from build123d import *

# Parameters (mm, degrees)
F0_R     = 10.428739
F1_DEPTH = 30


with BuildPart() as f1:
    # F0 (on Front) → F1 (new body)
    with BuildSketch(Plane.XZ):
        Polygon((-53.313535, -23.252012), (-53.313535, -43.252012), (16.686465, -43.252012), (16.686465, -28.252012), (25.202147, -21.013682), (15.48742, -9.584593), (5.770595, -17.843895), (2.121453, -13.550788), (13.550542, -3.83606), (2.27239, 9.432352), (-8.335778, 0.415407), (-18.335778, 0.415407), (-18.335778, -9.584593), (-23.335778, -9.584593), (-23.335778, 0.415407), (-43.335778, 0.415407), (-43.335778, -19.584593), align=None)
        with Locations((-20.813535, -28.252012)):
            Circle(F0_R, mode=Mode.SUBTRACT)
    extrude(amount=F1_DEPTH)


solid = f1.part
CAD build for the part. Positions are in the model's coordinates, mm. A direction names the side the tool comes from. Round coordinates to 2 decimals unless told otherwise and drop trailing zeros. Write each loop counter-clockwise with the first axis right and the second up, starting at its lowest first coordinate (ties: lowest second). Pieces come first, ordered by that corner, then holes.
(1) Slice it at A-A, the plane y = -16.5. Write the cut outline in (x, z).
(2) Drop flat-ended pins along their axis: P1, Ø7.5, axis at y = -19.5, z = -34.5, coming from the +X side; P2, Ø16, axis at x = -34, y = -11.5, coming from the +Z side; P3, Ø1.5, axis at x = 12.5, y = -10, coming from the +Z side. Give the stop position or say it passes through.
(3) Slice it at B-B, the plane z = -11. Write the cut outline in (x, y), and give its area (3 significant figures).
(4) Slice it at C-C, the plane x = -22.5. Write the cut outline in (y, z).
(5) Slice it at D-D, the plane x = -33.5. Write the cut outline in (y, z), and give its area (3 significant figures).
(6) Mould opens along Z. For faces 1 (the face through (-33, -15, 0.415)), 2 (the face through (-23.336, -15, -5)), 3 (the face through (-28.5, -14.79, -21.204)) say: pulls with the +Z half, pulls with the -Z half, needs draft (parallel to the pull), parting line crosses it, or undercut.
(7) Probe line 1 along X through (y, z) = (-18, -30.5); line 2 along X through (y, z) = (-14, -32.5); line 3 along Z through (x, y) = (10, -27.75). List the from-to ranges inside material, lowest first.
(8) 3-axis set-ups, long thin cutter, end or side, ignore diameter. For faces 4 (the face through (3.972, -14.79, -15.727)), 5 (the face through (-18.336, -15, -5)), 6 (the face through (16.686, -15, -36)), 7 (the face through (-13, -15, 0.415)): which of +Z, -Z, +X, -X, +Y, -Y reach the whole face in a straight line?
From the geometry:
1. outline: (-53.31, -43.25) - (16.69, -43.25) - (16.69, -28.25) - (25.2, -21.01) - (15.49, -9.58) - (5.77, -17.84) - (2.12, -13.55) - (13.55, -3.84) - (2.27, 9.43) - (-8.34, 0.42) - (-18.34, 0.42) - (-18.34, -9.58) - (-23.34, -9.58) - (-23.34, 0.42) - (-43.34, 0.42) - (-43.34, -19.58) - (-53.31, -23.25) - close; hole circle Ø20.86 at (-20.81, -28.25)
2. P1: stops at x = 16.69
2. P2: stops at z = 0.42
2. P3: stops at z = -1.72
3. outline: (-43.34, -30) - (5.12, -30) - (5.12, 0) - (-43.34, 0) - close; (13.82, -30) - (16.69, -30) - (16.69, 0) - (13.82, 0) - close
3. area: 1,540 mm2
4. outline: (-30, -43.25) - (0, -43.25) - (0, -38.54) - (-30, -38.54) - close; (-30, -17.96) - (0, -17.96) - (0, -9.58) - (-30, -9.58) - close
5. outline: (-30, -43.25) - (0, -43.25) - (0, 0.42) - (-30, 0.42) - close
5. area: 1,310 mm2
6. face 1: pulls with the +Z half
6. face 2: needs draft
6. face 3: undercut
7. line 1: x = -53.31 to -31, -10.63 to 16.69
7. line 2: x = -53.31 to -30.34, -11.29 to 16.69
7. line 3: z = -43.25 to -14.25, -6.85 to 0.34
8. face 4: +Y, -Y
8. face 5: +Z, +Y, -Y
8. face 6: -Z, +X, +Y, -Y
8. face 7: +Z, -X, +Y, -Y
